Autodesk Fusion 360 part; units mm, degrees
sketch "Sketch1" plane through (0, 0, 0) normal (0, 0, 1) x (1, 0, 0)
  line L0 (0, 0) -> (32.8, 0)
  line L1 (32.8, 0) -> (32.8, 2)
  line L2 (32.8, 2) -> (0, 2)
  line L3 (0, 2) -> (0, 0)
  line L4 (32.8, 0) -> (27.8, 0)
  line L5 (27.8, 0) -> (27.8, 23)
  line L6 (27.8, 23) -> (32.8, 23)
  line L7 (32.8, 23) -> (32.8, 0)
  line L8 (27.8, 23) -> (77.8, 23)
  line L9 (77.8, 23) -> (77.8, 21)
  line L10 (77.8, 21) -> (27.8, 21)
  line L11 (27.8, 21) -> (27.8, 23)
  dimension "d1" = 32.8
  dimension "d2" = 2
  dimension "d3" = 5
  dimension "d4" = 23
  dimension "d5" = 50
  dimension "d6" = 2
extrude "Extrude1" add sketch "Sketch1" along normal blind 55
sketch "Sketch2" plane through (0, 0, 0) normal (0, -1, 0) x (1, 0, 0)
  line L0 (0, 0) -> (32.8, 0)
  line L1 (32.8, 0) -> (32.8, 55)
  line L2 (32.8, 55) -> (0, 55)
  line L3 (0, 55) -> (0, 0)
  line L4 (12, 55) -> (12, 0) construction
  line L5 (0, 27.5) -> (32.8, 27.5) construction
  circle A0 centre (12, 47.5) radius 1.6
  circle A1 centre (12, 37.5) radius 1.6
  circle A2 centre (12, 17.5) radius 1.6
  circle A3 centre (12, 7.5) radius 1.6
  dimension "d10" = 3.2
  dimension "d11" = 3.2
  dimension "d12" = 3.2
  dimension "d13" = 3.2
  dimension "d14" = 10
  dimension "d15" = 10
  dimension "d17" = 10
  dimension "d19" = 10
  dimension "d30" = 12
extrude "Extrude2" cut sketch "Sketch2" against normal blind 25 contours A0 | A1 | A2 | A3
fillet "Fillet1" radius 2 1 edges at (32.8, 0, 27.5)
fillet "Fillet2" radius 2 1 edges at (27.8, 23, 27.5)
sketch "Sketch3" plane through (0, 21, 0) normal (0, -1, 0) x (1, 0, 0)
  line L0 (32.8, 0) -> (77.8, 0)
  line L1 (77.8, 0) -> (77.8, 55)
  line L2 (77.8, 55) -> (32.8, 55)
  line L3 (32.8, 55) -> (32.8, 0)
  line L4 (60.8, 55) -> (60.8, 0) construction
  line L5 (77.8, 27.5) -> (32.8, 27.5) construction
  circle A0 centre (60.8, 27.5) radius 5
  dimension "d26" = 28
  dimension "d27" = 10
extrude "Extrude3" cut sketch "Sketch3" against normal blind 15 contours A0
equation "bodyScrew = 3.2 mm"
equation "d10 = bodyScrew"
equation "d11 = bodyScrew"
equation "d12 = bodyScrew"
equation "d13 = bodyScrew"
Work out the finished part from the listing and answer in its coordinate system (mm). A direction names the side the tool comes from. Round coordinates to 2 decimals unless told otherwise and drop trailing zeros. Write each loop counter-clockwise with the first axis right and the second up, starting at its lowest first coordinate (ties: lowest second). Pieces come first, ordered by that corner, then holes. Notation, with made-up numbers: (28, -6.5) - (77, -6.5) arc R22 cw to (77, 13.5) - close; hole circle Ø10 at (11.25, 29.5). An arc over 180 degrees is marked (long way). Answer in a Markdown table with one row per item. Add a question column.
1. For faces 4 (the cylindrical face through (10.73, 0.99, 36.53)), 5 (the flat face through (55.6, 21, 27.1)), 6 (the flat face through (14, 2, 27)), determine the directions among +Z, -Z, +X, -X, +Y, -Y from which every point of the face is accessible in a straight line to the end or side of a thin tool.
2. A cutting plane is placed at C-C, the plane y = 11. Determine the outline of the cut face in (x, z), and give its area (3 significant figures).
3. A cutting plane is placed at A-A, the plane z = 27.5. Determine the outline of the cut face in (x, y), and give its area (3 significant figures).
4. The mould has two halves that part along X. Classify faces 1 (the flat face through (27.8, 11, 27)), 2 (the cylindrical face through (10.82, 0.99, 18.58)), 3 (the cylindrical face through (32.2, 0.57, 27.88)): +X half, -X half, draft (parallel to the pull), parting line (faces both ways), or undercut.
5. A cutting plane is placed at D-D, the plane z = 17.5. Determine the outline of the cut face in (x, y).
6. A cutting plane is placed at B-B, the plane z = 10.5. Determine the outline of the cut face in (x, y).
7. Find the intervals of material crossed by line 1 along Z through (x, y) = (12, 0.6); line 2 along Y through (x, z) = (65, 42); line 3 along X through (y, z) = (17, 40.5), in increasing order. Write a range as from..to.
8. Given pin 1 (6 mm diameter, centred on x = 61.5, z = 38, fed in from -Y); pin 2 (5 mm diameter, centred on x = 37.5, y = 3, fed in from -Z); pin 3 (8 mm diameter, centred on y = 4, z = 32.5, fed in from +X); pin 4 (5 mm diameter, centred on y = 17.5, z = 23.5, fed in from -X), each flat-ended and moving along its own axis, determine where each tip first touches the part or whether it passes through.
Worked out:
| question | item | result |
|---|---|---|
| 1 | face 4 | +Y, -Y |
| 1 | face 5 | +Z, -Z, +X, -Y |
| 1 | face 6 | +Z, -Z, -X, +Y |
| 2 | outline | (27.8, 0) - (32.8, 0) - (32.8, 55) - (27.8, 55) - close |
| 2 | area | 275 mm^2 |
| 3 | outline | (0, 0) - (30.8, 0) arc R2 ccw to (32.8, 2) - (32.8, 21) - (55.8, 21) - (55.8, 23) - (29.8, 23) arc R2 ccw to (27.8, 21) - (27.8, 2) - (0, 2) - close; (65.8, 21) - (77.8, 21) - (77.8, 23) - (65.8, 23) - close |
| 3 | area | 239 mm^2 |
| 4 | face 1 | -X half |
| 4 | face 2 | undercut |
| 4 | face 3 | +X half |
| 5 | outline | (0, 0) - (10.4, 0) - (10.4, 2) - (0, 2) - close; (13.6, 0) - (30.8, 0) arc R2 ccw to (32.8, 2) - (32.8, 21) - (77.8, 21) - (77.8, 23) - (29.8, 23) arc R2 ccw to (27.8, 21) - (27.8, 2) - (13.6, 2) - close |
| 6 | outline | (0, 0) - (30.8, 0) arc R2 ccw to (32.8, 2) - (32.8, 21) - (77.8, 21) - (77.8, 23) - (29.8, 23) arc R2 ccw to (27.8, 21) - (27.8, 2) - (0, 2) - close |
| 7 | line 1 | 0..5.9, 9.1..15.9, 19.1..35.9, 39.1..45.9, 49.1..55 |
| 7 | line 2 | 21..23 |
| 7 | line 3 | 27.8..32.8 |
| 8 | pin 1 | y = 21 |
| 8 | pin 2 | through |
| 8 | pin 3 | x = 32.8 |
| 8 | pin 4 | x = 27.8 |
